Geometry check sheet. Reference: the model listing, model coordinates, mm. Round coordinates to 2 decimals unless told otherwise and drop trailing zeros. Loops run counter-clockwise (first coordinate to the right, second up) from the corner with the lowest first, then second, coordinate; pieces in that order, holes last. Notation, with made-up numbers: (26, 64.25) - (56, 64.25) arc R28 cw to (56, 85.25) - close; hole circle Ø6 at (83.5, -29). An arc over 180 degrees is marked (long way). Answer in a Markdown table with one row per item. Add a question column.
```python
from build123d import *

# Parameters (mm, degrees)
SKETCH_1_R      = 3
EXTRUDE_1_DEPTH = 8


with BuildPart() as part:
    # 草图1 → 凸台-拉伸1 (new body)
    with BuildSketch(Plane.XY.offset(8)):
        with BuildLine():
            Line((12, -36), (12, 0))
            ThreePointArc((12, 0), (0, 12), (-12, 0))
            Line((-12, 0), (-12, -36))
            ThreePointArc((-12, -36), (0, -48), (12, -36))
        make_face()
        with Locations((0, -36)):
            Circle(SKETCH_1_R, mode=Mode.SUBTRACT)
        Circle(SKETCH_1_R, mode=Mode.SUBTRACT)
    extrude(amount=-EXTRUDE_1_DEPTH)


solid = part.part
```
Q1. Release check for a two-part mould opening along Y. For faces 1 (the cylindrical face through (0, -48, 4)), 2 (the cylindrical face through (0, 12, 4)), 3 (the cylindrical face through (0, -33, 4)), 4 (the flat face through (12, -18, 4)) record: +Y half, -Y half, draft (parallel to the pull), parting line (faces both ways), or undercut.
Q2. Scan lines: line 1 (Y direction, x = 0, z = 5.5); line 2 (Y direction, x = -2.75, z = 7.25); line 3 (X direction, y = 2.5, z = 6.25). Record each from-to range of solid material in increasing order. Write a range as from..to.
Q3. Cross-section at A-A, the plane x = 0. Enter the section's corners in (y, z), plus the area to 3 significant figures.
Q4. Cross-section at D-D, the plane x = -6.75. Enter the section's corners in (y, z), plus the area to 3 significant figures.
Q5. Cross-section at C-C, the plane y = -43. Enter the section's corners in (x, z), plus the area to 3 significant figures.
Q6. Depth check by flat-ended pin: P1, Ø1.5, axis at x = -1.5, z = 7, coming from the +Y side; P2, Ø1, axis at x = -8.5, z = 6, coming from the -Y side. Enter the tip coordinate at first touch or a pass-through.
Q7. Cross-section at B-B, the plane y = 2. Enter the section's corners in (x, z).
Check sheet entries:
| question | item | result |
|---|---|---|
| 1 | face 1 | -Y half |
| 1 | face 2 | +Y half |
| 1 | face 3 | undercut |
| 1 | face 4 | draft |
| 2 | line 1 | -48..-39, -33..-3, 3..12 |
| 2 | line 2 | -47.68..-37.2, -34.8..-1.2, 1.2..11.68 |
| 2 | line 3 | -11.74..-1.66, 1.66..11.74 |
| 3 | outline | (-48, 0) - (-39, 0) - (-39, 8) - (-48, 8) - close; (-33, 0) - (-3, 0) - (-3, 8) - (-33, 8) - close; (3, 0) - (12, 0) - (12, 8) - (3, 8) - close |
| 3 | area | 384 mm² |
| 4 | outline | (-45.92, 0) - (9.92, 0) - (9.92, 8) - (-45.92, 8) - close |
| 4 | area | 447 mm² |
| 5 | outline | (-9.75, 0) - (9.75, 0) - (9.75, 8) - (-9.75, 8) - close |
| 5 | area | 156 mm² |
| 6 | P1 | y = 11.98 |
| 6 | P2 | y = -44.94 |
| 7 | outline | (-11.83, 0) - (-2.24, 0) - (-2.24, 8) - (-11.83, 8) - close; (2.24, 0) - (11.83, 0) - (11.83, 8) - (2.24, 8) - close |
